Input: part model. Units: mm. Frame: model coordinates. A direction names the side the tool comes from. Round coordinates to 2 decimals unless told otherwise and drop trailing zeros. Loops run counter-clockwise (first coordinate to the right, second up) from the corner with the lowest first, then second, coordinate; pieces in that order, holes last. Notation, with made-up numbers: (25, -14) - (51, -14) arc R16 cw to (51, -3) - close; hole circle Ø4 at (60, -19.5). An arc over 180 degrees is marked (long way). Use CSV: the item, a comma, the result in double quotes. Start each with the question number.
1. Pin query (flat end, axial travel): P1, Ø5, axis at x = 0, z = 31.75, coming from the -Y side. Return the tip coordinate at first contact, or that it passes through.
2. Cut plane C-C (z = -12). Return loops of the section in (x, y) (3 decimals).
3. Pull-direction query (X, two-part tool) for faces 3 (the flat face through (34.925, 0, 0)), 4 (the cylindrical face through (31.23, -0.03, -21.22)), 5 (the flat face through (0, 0, 34.925)); classes: +X half, -X half, draft (parallel to the pull), parting line (faces both ways), or undercut.
4. Cut plane A-A (z = -31.75). Return loops of the section in (x, y) (1 decimal).
5. Material intervals for probe 1 along X at (y, z) = (-1.05, -31.75) (1 decimal); probe 2 along Z at (x, y) = (4.5, -2.1) (3 decimals); probe 3 along X at (y, z) = (-0.6, 23) (3 decimals), sorted ascending. Write a range as from..to.
6. Access query for faces 1 (the flat face through (0, 0, -19.05)), 2 (the flat face through (0, 0, -34.925)). Directions: +Z, -Z, +X, -X, +Y, -Y. A direction counts if a zero-diameter tool reaches every point of the face in a straight line with its end or side. Return the directions, or none.
7. Cut plane B-B (x = 0). Give the number of separate pieces and of enclosed holes in the cut face, and give its area (3 significant figures).
```python
from build123d import *

# Parameters (mm, degrees)
SKETCH1_W                    = 69.85
SKETCH1_H                    = 69.85
BOSS_EXTRUDE1_DEPTH          = 2.38125
CUT_EXTRUDE1_REACH           = 51.62
SKETCH2_W                    = 38.1
SKETCH2_H                    = 38.1
F_4_40_TAPPED_HOLE1_D        = 2.2606
F_1_8_0_125_DIAMETER_HOLE1_D = 3.175


with BuildPart() as part:
    # Sketch1 → Boss-Extrude1 (new, symmetric)
    with BuildSketch(Plane(origin=(0, 0, 0), x_dir=(1, 0, 0), z_dir=(0, 1, 0))):
        Rectangle(SKETCH1_W, SKETCH1_H)
    extrude(amount=BOSS_EXTRUDE1_DEPTH, both=True)

    # Sketch2 → Cut-Extrude1 (cut, up to next)
    with BuildSketch(Plane(origin=(0, 2.38125, 0), x_dir=(1, 0, 0), z_dir=(0, 1, 0)), mode=Mode.PRIVATE) as cut_extrude1_sk1:
        Rectangle(SKETCH2_W, SKETCH2_H)
    cut_extrude1_tool1 = extrude(cut_extrude1_sk1.sketch, amount=-CUT_EXTRUDE1_REACH, mode=Mode.PRIVATE) & part.part
    add(cut_extrude1_tool1.solids().sort_by_distance((0, 2.38125, 0))[0], mode=Mode.SUBTRACT)

    # #4-40 Tapped Hole1 (through all)
    with Locations(Plane(origin=(0, 2.38125, 0), x_dir=(1, 0, 0), z_dir=(0, 1, 0))):
        with Locations((-31.75, 22.225), (31.75, 22.225)):
            f_4_40_tapped_hole1 = Hole(F_4_40_TAPPED_HOLE1_D / 2)

    # 1/8 (0.125) Diameter Hole1 (through all)
    with Locations(Plane(origin=(0, 2.38125, 0), x_dir=(1, 0, 0), z_dir=(0, 1, 0))):
        with Locations((-29.21, 31.75), (29.21, 31.75), (0, -31.75)):
            Hole(F_1_8_0_125_DIAMETER_HOLE1_D / 2)

    # Mirror1: #4-40 Tapped Hole1 across plane
    add(f_4_40_tapped_hole1.mirror(Plane.XY), mode=Mode.SUBTRACT)


solid = part.part
```
Established:
1,P1,"stops at y = -2.38"
2,outline,"(-34.925, -2.381) - (-19.05, -2.381) - (-19.05, 2.381) - (-34.925, 2.381) - close; (19.05, -2.381) - (34.925, -2.381) - (34.925, 2.381) - (19.05, 2.381) - close"
3,face 3,"+X half"
3,face 4,"undercut"
3,face 5,"draft"
4,outline,"(-34.9, -2.4) - (-30.8, -2.4) - (-30.8, 2.4) - (-34.9, 2.4) - close; (-27.6, -2.4) - (27.6, -2.4) - (27.6, 2.4) - (-27.6, 2.4) - close; (30.8, -2.4) - (34.9, -2.4) - (34.9, 2.4) - (30.8, 2.4) - close"
5,probe 1,"x = -34.9..-30.8, -27.6..27.6, 30.8..34.9"
5,probe 2,"z = -34.925..-19.05, 19.05..34.925"
5,probe 3,"x = -34.925..-32.573, -30.927..30.927, 32.573..34.925"
6,face 1,"+Y, -Y"
6,face 2,"-Z, +X, -X, +Y, -Y"
7,separate pieces,"3"
7,enclosed holes,"0"
7,area,"136 mm2"
